Part model, mm, in its own coordinate system. Round coordinates to 2 decimals unless told otherwise and drop trailing zeros. Loops run counter-clockwise (first coordinate to the right, second up) from the corner with the lowest first, then second, coordinate; pieces in that order, holes last.
from build123d import *

# Parameters (mm, degrees)
SKETCH_1_R               = 15.91549431
EXTRUDE_1_DEPTH          = 15
SKETCH_2_R               = 4.1
CUT_EXTRUDE_5_DEPTH      = 15
SKETCH_5_RX              = 2
SKETCH_5_RY              = 1
CUT_EXTRUDE_6_DEPTH      = 15
PATTERN_CIRCULAR_2_COUNT = 18


with BuildPart() as part:
    # Эскиз1 → Бобышка-Вытянуть1 (new body)
    with BuildSketch(Plane.XY):
        Circle(SKETCH_1_R)
    extrude(amount=EXTRUDE_1_DEPTH)

    # Эскиз2 → Вырез-Вытянуть5 (cut)
    with BuildSketch(Plane.XY.offset(15)):
        Circle(SKETCH_2_R)
    extrude(amount=-CUT_EXTRUDE_5_DEPTH, mode=Mode.SUBTRACT)

    # Эскиз5 → Вырез-Вытянуть6 (cut)
    with BuildSketch(Plane.XY.offset(15)):
        with Locations(Location((0.082802385, 15.915278914), (0, 0, 89.70191007))):
            Ellipse(SKETCH_5_RX, SKETCH_5_RY)
    cut_extrude_6 = extrude(amount=-CUT_EXTRUDE_6_DEPTH, mode=Mode.SUBTRACT)

    # Круговой массив2: Вырез-Вытянуть6 ×18 about axis
    pattern_circular_2_axis = Axis((0, 0, 0), (0, 0, 1))
    for i in range(1, PATTERN_CIRCULAR_2_COUNT):
        add(cut_extrude_6.rotate(pattern_circular_2_axis, i * 360 / PATTERN_CIRCULAR_2_COUNT), mode=Mode.SUBTRACT)


solid = part.part
1) Drop flat-ended pins along their axis: pin 1 Ø1.5 at (x, z) = (11, 9.5) entering from +Y; pin 2 Ø5 at (x, z) = (11.5, 11.5) entering from +Y; pin 3 Ø1.5 at (y, z) = (12.5, 13) entering from +X. Give the stop position or say it passes through.
Values:
pin 1: stops at y = 11.47
pin 2: stops at y = 13.13
pin 3: stops at x = 9.51
2) Mould opens along Y. For faces 1 (the face through (2.87, 15.655, 7.395)), 2 (the face through (2.66, -15.69, 7.4)), 3 (the face through (-0.534, 4.065, 7.605)), 4 (the face through (3.3, -3.3, 15)) say: released by +Y, released by -Y, zero draft, split by the parting line, or undercut.
Values:
face 1: released by +Y
face 2: released by -Y
face 3: undercut
face 4: zero draft
3) Wall check: line 1 along Y through (x, z) = (0, 4); line 2 along Y through (x, z) = (-9, 10); line 3 along Y through (x, z) = (12.5, 1.5). Give the ranges that are in metal, low to high.
Values:
line 1: y = -13.92 to -4.1, 4.1 to 13.92
line 2: y = -13.13 to -11.97, -10.61 to 10.64, 12.31 to 13.13
line 3: y = -9.85 to -8.33, -6.72 to 6.61, 8.11 to 9.85
4) Slice it at A-A, the plane y = 0. Give the cut face in (x, z).
Values:
outline: (-15.92, 0) - (-4.1, 0) - (-4.1, 15) - (-15.92, 15) - close; (4.1, 0) - (15.92, 0) - (15.92, 15) - (4.1, 15) - close
